Design review of the part built by this model. Coordinates are the model's own, in mm. Face numbers are marked on the shaded views. Coordinates: 2 decimals unless noted, no trailing zeros. Write each loop counter-clockwise with the first axis right and the second up, starting at its lowest first coordinate (ties: lowest second). Pieces come first, ordered by that corner, then holes.
Q1. For probe 1 along Y at (x, z) = (0, 433.5); probe 2 along Z at (x, y) = (-164, -180.5); probe 3 along X at (y, z) = (240, 62.5), list the stretches that pass through material, from the lowest coordinate up.
Q2. Take a section at A-A (y = 0). Give the boundary of the cut face in (x, z), and give its area (3 significant figures).
Q3. Take a section at B-B (z = 350.5). Give the boundary of the cut face in (x, y).
Q4. Take a section at D-D (y = 235). Give the boundary of the cut face in (x, z), and give its area (3 significant figures).
Q5. Mouldability with a two-part tool opening along Y and no side actions: class the marked faces 1 and 2 as pulls with the +Y half, pulls with the -Y half, needs draft (parallel to the pull), parting line crosses it, or undercut.
Q6. Insertion check: pin 1 (2 mm diameter, centred on x = 178.5, y = 38.5, fed in from -Z); pin 2 (20.5 mm diameter, centred on x = 0, y = 0, fed in from +Z); pin 3 (15 mm diameter, centred on x = -240, z = 129.5, fed in from -Y). Each pin has a flat end and moves straight along its axis. Give the tip position at first contact, or say it passes through.
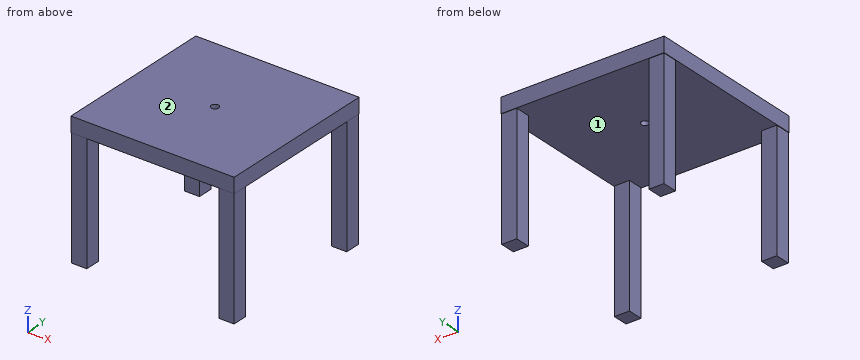
```python
from build123d import *

# Parameters (mm, degrees)
F0_W     = 50.8
F0_H     = 50.8
F1_DEPTH = 400.05
F2_W     = 549.275
F2_H     = 549.275
F2_W_2   = 50.8
F2_H_2   = 50.8
F3_DEPTH = 50.8
F4_R     = 12.7
F5_DEPTH = 450.851


with BuildPart() as f1:
    # F0 (on Top) → F1 (new body)
    with BuildSketch(Plane.XY):
        with Locations((-247.65, 247.65)):
            Rectangle(F0_W, F0_H)
    extrude(amount=F1_DEPTH)



with BuildPart() as f1b:
    # F0 (on Top) → F1, piece 2 (new body)
    with BuildSketch(Plane.XY):
        with Locations((247.65, 247.65)):
            Rectangle(F0_W, F0_H)
    extrude(amount=F1_DEPTH)


with BuildPart() as f1c:
    # F0 (on Top) → F1, piece 3 (new body)
    with BuildSketch(Plane.XY):
        with Locations((-247.65, -247.65)):
            Rectangle(F0_W, F0_H)
    extrude(amount=F1_DEPTH)


with BuildPart() as f1d:
    # F0 (on Top) → F1, piece 4 (new body)
    with BuildSketch(Plane.XY):
        with Locations((247.65, -247.65)):
            Rectangle(F0_W, F0_H)
    extrude(amount=F1_DEPTH)


with BuildPart() as f1_1:
    add(f1.part)

    add(f1b.part)  # F3 merges F1b

    add(f1c.part)  # F3 merges F1c

    add(f1d.part)  # F3 merges F1d
    # F2 (on face) → F3 (join)
    with BuildSketch(Plane.XY.offset(400.05)):
        Rectangle(F2_W, F2_H)
        with Locations((-247.65, -247.65)):
            Rectangle(F2_W_2, F2_H_2, mode=Mode.SUBTRACT)
        with Locations((-247.65, -247.65)):
            Rectangle(F2_W_2, F2_H_2)
    extrude(amount=F3_DEPTH)

    # F4 (on face) → F5 (cut, through all)
    with BuildSketch(Plane.XY.offset(450.85)):
        Circle(F4_R)
    extrude(amount=-F5_DEPTH, mode=Mode.SUBTRACT)


solid = f1_1.part
```
Response:
1. probe 1: y = -274.64 to -12.7, 12.7 to 274.64
1. probe 2: z = 400.05 to 450.85
1. probe 3: x = -273.05 to -222.25, 222.25 to 273.05
2. outline: (-274.64, 400.05) - (-12.7, 400.05) - (-12.7, 450.85) - (-274.64, 450.85) - close; (12.7, 400.05) - (274.64, 400.05) - (274.64, 450.85) - (12.7, 450.85) - close
2. area: 26,600 mm2
3. outline: (-273.05, -273.05) - (-222.25, -273.05) - (-222.25, -222.25) - (-273.05, -222.25) - close; (-273.05, 222.25) - (-222.25, 222.25) - (-222.25, 273.05) - (-273.05, 273.05) - close; (222.25, -273.05) - (273.05, -273.05) - (273.05, -222.25) - (222.25, -222.25) - close; (222.25, 222.25) - (273.05, 222.25) - (273.05, 273.05) - (222.25, 273.05) - close
4. outline: (-274.64, 400.05) - (-273.05, 400.05) - (-273.05, 0) - (-222.25, 0) - (-222.25, 400.05) - (222.25, 400.05) - (222.25, 0) - (273.05, 0) - (273.05, 400.05) - (274.64, 400.05) - (274.64, 450.85) - (-274.64, 450.85) - close
4. area: 68,500 mm2
5. face 1: undercut
5. face 2: needs draft
6. pin 1: stops at z = 400.05
6. pin 2: passes through
6. pin 3: stops at y = -273.05
